Geometry check sheet. Reference: the model listing, model coordinates, mm. Face numbers are marked on the shaded views. A direction names the side the tool comes from. Give positions to 0.01 mm unless a question says otherwise; leave off trailing zeros. Loops run counter-clockwise (first coordinate to the right, second up) from the corner with the lowest first, then second, coordinate; pieces in that order, holes last. Notation, with made-up numbers: (65, 24.25) -> (115, 24.25) arc R14 ccw to (115, 46.25) -> close; hole circle Ø7 at (31.25, 57). An arc over 180 degrees is marked (long way). Write item = value, one per line.
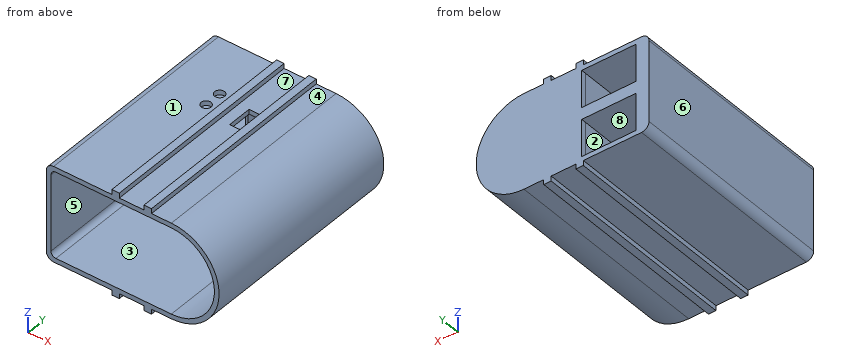
Autodesk Inventor part; units mm, degrees
ref_plane "Work Plane1" through (0, 85, 0) normal (0, 1, 0) x (1, 0, 0)
ref_plane "YZ Plane" through (0, 0, 0) normal (1, 0, 0) x (0, 1, 0)
ref_plane "XZ Plane" through (0, 0, 0) normal (0, 1, 0) x (-1, 0, 0)
sketch "Sketch1" plane through (0, 0, 0) normal (0, 1, 0) x (-1, 0, 0)
  line L0 (35.4, 17.4) -> (35.4, -17.4)
  line L1 (35.4, -17.4) -> (-13.2013, -17.4)
  arc A0 (-13.2013, 17.4) -> (-13.2013, -17.4) centre (-13.2013, 0) ccw
  line L2 (-13.2013, 17.4) -> (35.4, 17.4)
  line L3 (37.3, -19.3) -> (37.3, 19.3)
  line L4 (37.3, 19.3) -> (-13.2013, 19.3)
  arc A1 (-13.2013, 19.3) -> (-13.2013, -19.3) centre (-13.2013, 0) ccw
  line L5 (-13.2013, -19.3) -> (37.3, -19.3)
  point P0 (0, 0)
  point P1 (-13.2013, 0)
  point P2 (0, 0)
  point P3 (-12.8411, -36.7096)
  point P4 (-12.8411, -7.716)
  point P5 (-24.0253, -72.4098)
extrude "Extrusion1" add sketch "Sketch1" along normal blind 83
ref_plane "Work Plane1" through (0, 85, 0) normal (0, 1, 0) x (1, 0, 0)
sketch "Sketch2" plane through (0, 85, 0) normal (0, 1, 0) x (1, 0, 0)
  line L0 (-37.3, 19.3) -> (-37.3, -19.3)
  line L1 (-37.3, -19.3) -> (13.2013, -19.3)
  arc A0 (13.2013, -19.3) -> (13.2013, 19.3) centre (13.2013, 0) ccw
  line L2 (13.2013, 19.3) -> (-37.3, 19.3)
  point P0 (0, 0)
  point P1 (0, 0)
  point P2 (13.2013, 0)
  point P3 (0, 0)
  point P4 (14.0497, 95.3418)
  point P5 (14.0497, 124.3354)
  point P6 (2.8654, 59.6417)
extrude "Extrusion2" add sketch "Sketch2" against normal up to surface (2 mm away)
fillet "Fillet1" radius 3 3 edges at (-37.3, 41.5, -19.3) (-37.3, 84, -19.3) (-37.3, 42.5, 19.3)
fillet "Fillet2" radius 2 2 edges at (-35.4, 41.5, -17.4) (-35.4, 41.5, 17.4)
sketch "Sketch3" plane through (13.2013, 0, -19.3) normal (0, 0, -1) x (-1, 0, 0)
  line L0 (0, 85) -> (47.5013, 85)
  line L1 (0, 0) -> (47.5013, 0)
  line L2 (8, 85) -> (11, 85)
  line L3 (11, 85) -> (11, 0)
  line L4 (11, 0) -> (8, 0)
  line L5 (8, 0) -> (8, 85)
  line L6 (0, 0) -> (0, 85)
  point P0 (8, 0)
  point P1 (11, 85)
  dimension "d28" = 3
  dimension "d29" = 8
extrude "Extrusion5" add sketch "Sketch3" along normal blind 2 contours L0 L3 L1 L5
sketch "Sketch8" plane through (-34.3, 0, -19.3) normal (0, 0, -1) x (-1, 0, 0)
  line L0 (0, 85) -> (-47.5013, 85)
  line L1 (-36.5013, 0) -> (0, 0)
  line L2 (-26.5013, 85) -> (-23.5013, 85)
  line L3 (-23.5013, 85) -> (-23.5013, 0)
  line L4 (-23.5013, 0) -> (-26.5013, 0)
  line L5 (-26.5013, 0) -> (-26.5013, 85)
  line L6 (-36.5013, 0) -> (-36.5013, 85)
  point P0 (-34.3, 0)
  point P1 (-26.5013, 0)
  dimension "d34" = 10
  dimension "d35" = 3
extrude "Extrusion6" add sketch "Sketch8" along normal blind 2 contours L3 L1 L5 L0
sketch "Sketch9" plane through (13.2013, 0, 19.3) normal (0, 0, 1) x (1, 0, 0)
  line L0 (-47.5013, 85) -> (0, 85)
  line L1 (-46.6013, 0) -> (0, 0)
  line L2 (-11, 85) -> (-8, 85)
  line L3 (-8, 85) -> (-8, 0)
  line L4 (-8, 0) -> (-11, 0)
  line L5 (-11, 0) -> (-11, 85)
  line L6 (0, 0) -> (0, 85)
  point P0 (-13.2013, 0)
  point P1 (-11, 0)
  dimension "d38" = 8
  dimension "d39" = 3
extrude "Extrusion7" add sketch "Sketch9" along normal blind 2 contours L0 L3 L1 L5
sketch "Sketch10" plane through (-34.3, 0, 19.3) normal (0, 0, 1) x (1, 0, 0)
  line L0 (47.5013, 0) -> (0.9, 0)
  line L1 (23.5013, 85) -> (0, 85)
  line L2 (26.5013, 0) -> (23.5013, 0)
  line L3 (23.5013, 0) -> (23.5013, 85)
  line L4 (23.5013, 85) -> (26.5013, 85)
  line L5 (26.5013, 85) -> (26.5013, 0)
  line L6 (36.5013, 85) -> (36.5013, 0)
  point P0 (34.3, 0)
  point P1 (23.5013, 0)
  dimension "d42" = 10
  dimension "d43" = 3
extrude "Extrusion8" add sketch "Sketch10" along normal blind 2
sketch "Sketch14" plane through (13.2013, 83, 0) normal (0, -1, 0) x (1, 0, 0)
  line L0 (-46.6013, -17.4) -> (0, -17.4)
  line L1 (-45.348, -17.4) -> (-23.348, -17.4)
  line L2 (-23.348, -17.4) -> (-23.348, -2.4)
  line L3 (-23.348, -2.4) -> (-45.348, -2.4)
  line L4 (-45.348, -2.4) -> (-45.348, -17.4)
  line L5 (-46.348, -17.4) -> (-22.348, -17.4)
  line L6 (-22.348, -17.4) -> (-22.348, -1.4)
  line L7 (-22.348, -1.4) -> (-46.348, -1.4)
  line L8 (-46.348, -1.4) -> (-46.348, -17.4)
  point P0 (-13.2013, 0)
  point P1 (-23.348, -17.4)
  point P2 (-22.348, -17.4)
  dimension "d50" = 22
  dimension "d51" = 15
  dimension "d52" = 1
  dimension "d53" = 1
  dimension "d54" = 1
extrude "Extrusion11" add sketch "Sketch14" along normal blind 15 contours L8 L7 L6 L0 L2 L3 L4
sketch "Sketch16" plane through (-32.1466, 83, -17.4) normal (0, -1, 0) x (1, 0, 0)
  line L0 (0, 0) -> (22, 0)
  line L1 (22, 0) -> (22, 15)
  line L2 (22, 15) -> (0, 15)
  line L3 (0, 15) -> (0, 0)
  line L4 (0, 15) -> (22, 15)
  line L5 (22, 15) -> (22, 0)
  point P0 (32.1466, 17.4)
  dimension "d57" = 0
  dimension "d58" = 0
extrude "Extrusion12" cut sketch "Sketch16" against normal through all
sketch "Sketch19" plane through (13.2013, 83, 0) normal (0, -1, 0) x (1, 0, 0)
  line L0 (0, 17.4) -> (-46.6013, 17.4)
  line L1 (-23.348, 17.4) -> (-45.348, 17.4)
  line L2 (-45.348, 17.4) -> (-45.348, 2.4)
  line L3 (-45.348, 2.4) -> (-23.348, 2.4)
  line L4 (-23.348, 2.4) -> (-23.348, 17.4)
  line L5 (-22.348, 17.4) -> (-46.348, 17.4)
  line L6 (-46.348, 17.4) -> (-46.348, 1.4)
  line L7 (-46.348, 1.4) -> (-22.348, 1.4)
  line L8 (-22.348, 1.4) -> (-22.348, 17.4)
  line L9 (-46.348, -1.4) -> (-46.348, -17.4)
  point P0 (-13.2013, 0)
  point P1 (-22.348, 9.4)
  dimension "d68" = 15
  dimension "d69" = 22
  dimension "d70" = 1
  dimension "d71" = 1
  dimension "d72" = 1
  dimension "d73" = 0
extrude "Extrusion15" add sketch "Sketch19" along normal blind 15 contours L8 L7 L6 L0 L2 L3 L4
sketch "Sketch22" plane through (-32.1466, 83, 17.4) normal (0, -1, 0) x (1, 0, 0)
  line L0 (22, -15) -> (0, -15)
  line L1 (0, 0) -> (0, -15)
  line L2 (22, -15) -> (0, -15)
  line L3 (0, -15) -> (0, 0)
  line L4 (0, 0) -> (22, 0)
  line L5 (22, 0) -> (22, -15)
  point P0 (32.1466, -17.4)
extrude "Extrusion16" cut sketch "Sketch22" against normal through all
sketch "Sketch28" plane through (2.2013, 0, 19.3) normal (0, 0, 1) x (1, 0, 0)
  line L0 (-5.75, 61.5) -> (-1.25, 61.5)
  line L1 (-1.25, 61.5) -> (-1.25, 51.5)
  line L2 (-1.25, 51.5) -> (-5.75, 51.5)
  line L3 (-5.75, 51.5) -> (-5.75, 61.5)
  line L4 (-10, 0) -> (0, 0)
  line L5 (11, 0) -> (11, 85)
  point P0 (-2.2013, 0)
  point P1 (-3.5, 61.5)
  point P2 (-3.5, 51.5)
  dimension "d106" = 61.5
  dimension "d107" = 10
  dimension "d108" = 4.5
  dimension "d109" = 12.25
extrude "Extrusion22" cut sketch "Sketch28" against normal up to surface (1.9 mm away)
sketch "Sketch31" plane through (-34.3, 0, 19.3) normal (0, 0, 1) x (1, 0, 0)
  line L0 (23.5013, 85) -> (23.5013, 0)
  line L1 (0, 85) -> (23.5013, 85)
  point P0 (34.3, 0)
  point P1 (18.5013, 62)
  dimension "d124" = 5
  dimension "d125" = 23
hole "Hole1" at (-15.7987, 62, 19.3) direction (0, 0, -1) diameter 4 depth 1.9
pattern_linear "Rectangular Pattern1" count 2 spacing 7 along (0, -1, 0) of "Hole1"
properties part number "víko"
Item 1: Thickness scan on L1, parallel to Z at x = -26, y = 69.5; L2, parallel to X at y = 78.5, z = -3; L3, parallel to X at y = 71.5, z = 4.5. Record the ranges inside material, lowest first. Write a range as [from, to].
Answer:
L1 = [-19.3, -17.4], [-2.4, -1.4], [1.4, 2.4], [17.4, 19.3]
L2 = [-37.3, -35.4], [-33.15, -32.15], [-10.15, -9.15], [30.34, 32.27]
L3 = [-37.3, -35.4], [-33.15, -32.15], [-10.15, -9.15], [30.01, 31.97]
Item 2: Tool access check on the marked faces 1, 2, 3 and 4. Record the directions out of +Z, -Z, +X, -X, +Y, -Y that give a thin tool (end or side, any length) a straight path to the whole face; none if there is none.
Answer:
face_1 = +Z, -X, +Y, -Y
face_2 = +Y, -Y
face_3 = -Y
face_4 = +Z, +X, +Y, -Y
Item 3: Gauge pin test, flat ends, axial feed: pin 1 (10 mm diameter, centred on y = 47, z = 10, fed in from +X); pin 2 (4.5 mm diameter, centred on y = 79, z = 9, fed in from +X); pin 3 (3 mm diameter, centred on x = -15.8, y = 62, fed in from +Z). Record the tip position at first contact, or that the pin passes through.
Answer:
pin_1 = 31.84
pin_2 = 31.28
pin_3 = -17.4
Item 4: Section check B-B, the plane z = 0. Record the cut outline in (x, y).
Answer:
outline = (-37.3, 0) -> (-35.4, 0) -> (-35.4, 83) -> (30.6, 83) -> (30.6, 0) -> (32.5, 0) -> (32.5, 85) -> (-37.3, 85) -> close
Item 5: Draft check along Z on the marked faces 5, 6, 7 and 8. Enter one of: +Z half, -Z half, draft (parallel to the pull), parting line (faces both ways), or undercut.
Answer:
face_5 = undercut
face_6 = draft
face_7 = +Z half
face_8 = undercut
Item 6: Section check C-C, the plane y = 75. Give the number of separate pieces and of enclosed holes in the cut face, plus the area to 3 significant figures.
Answer:
separate_pieces = 1
enclosed_holes = 3
area = 497 mm^2
